Geometry: see drawing. Coordinates: mm, zero at the bounding-box minimum. Give positions to 0.01 mm unless a question says otherwise; leave off trailing zeros. Loops run counter-clockwise (first coordinate to the right, second up) from the corner with the lowest first, then second, coordinate; pieces in that order, holes last. Notation, with made-up numbers: (49.5, 79) -> (60.5, 79) arc R31 cw to (60.5, 103) -> close; hole circle Ø11 at (81, 61.5). An arc over 180 degrees is marked (long way). Return JSON: item names as keys, results as strings. Group by question number.
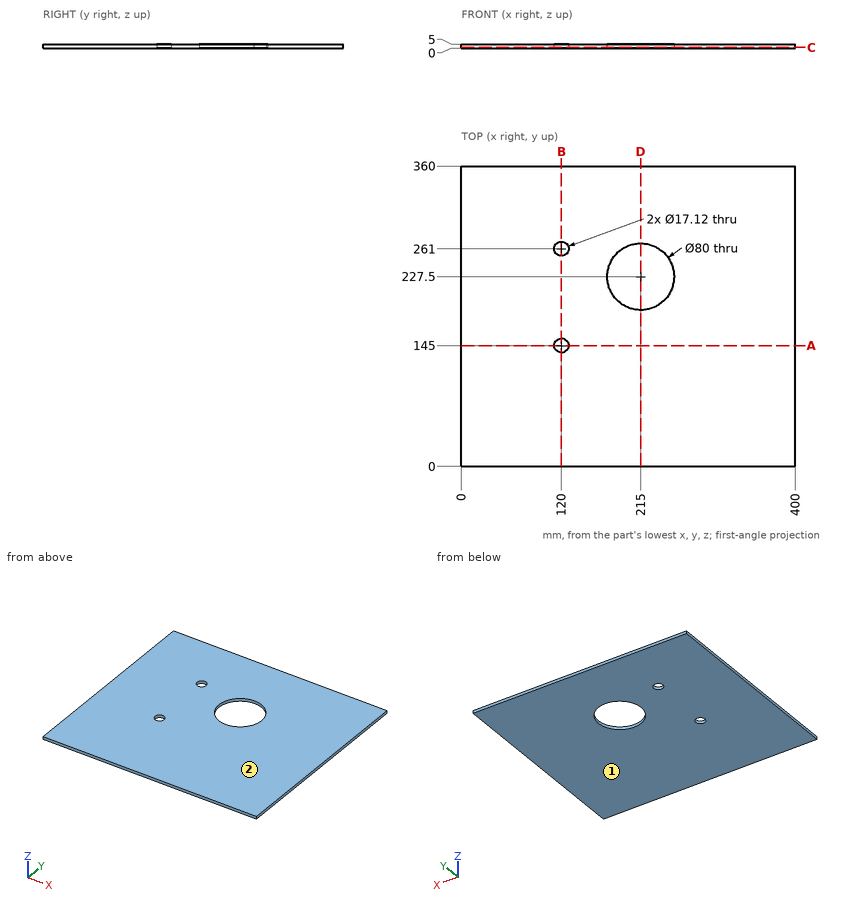
1) Cut plane B-B on x = 120. Return loops of the section in (y, z).
2) Contact query for a flat-ended pin moving along its axis: P1, Ø13.5, axis at x = 120, y = 145, coming from the +Z side. Output: stop coordinate, or through.
3) Material intervals for line 1 (Y direction, x = 120, z = 3.4); line 2 (X direction, y = 261, z = 2.15); line 3 (Y direction, x = 123.5, z = 0.45), sorted ascending.
4) Mould query, pull axis Z, two halves, no side actions, for the marked faces 1 and 2. Classes: released by +Z, released by -Z, zero draft, split by the parting line, or undercut.
5) Cut plane D-D on x = 215. Return loops of the section in (y, z), then the cut area to 3 significant figures.
6) Cut plane C-C on z = 0.9. Return loops of the section in (x, y).
7) Cut plane A-A on y = 145. Return loops of the section in (x, z), then the cut area to 3 significant figures.
Calculated:
{
 "1": {"outline": "(0, 0) -> (136.44, 0) -> (136.44, 5) -> (0, 5) -> close; (153.56, 0) -> (252.44, 0) -> (252.44, 5) -> (153.56, 5) -> close; (269.56, 0) -> (360, 0) -> (360, 5) -> (269.56, 5) -> close"},
 "2": {"P1": "through"},
 "3": {"line 1": "0 to 136.44, 153.56 to 252.44, 269.56 to 360", "line 2": "0 to 111.44, 128.56 to 193.14, 236.86 to 400", "line 3": "0 to 137.19, 152.81 to 253.19, 268.81 to 360"},
 "4": {"face 1": "released by -Z", "face 2": "released by +Z"},
 "5": {"outline": "(0, 0) -> (187.5, 0) -> (187.5, 5) -> (0, 5) -> close; (267.5, 0) -> (360, 0) -> (360, 5) -> (267.5, 5) -> close", "area": "1,400 mm2"},
 "6": {"outline": "(0, 0) -> (400, 0) -> (400, 360) -> (0, 360) -> close; hole circle Ø17.12 at (120, 145); hole circle Ø17.12 at (120, 261); hole circle Ø80 at (215, 227.5)"},
 "7": {"outline": "(0, 0) -> (111.44, 0) -> (111.44, 5) -> (0, 5) -> close; (128.56, 0) -> (400, 0) -> (400, 5) -> (128.56, 5) -> close", "area": "1,910 mm2"}
}
